from build123d import *

# Parameters (mm, degrees)
CROQUIS1_W                 = 195
CROQUIS1_H                 = 38
CROQUIS1_R                 = 1.625
SALIENTE_EXTRUIR1_DEPTH    = 3
CROQUIS8_W                 = 195
CROQUIS8_H                 = 3
SALIENTE_EXTRUIR5_DEPTH    = 5
CROQUIS9_W                 = 195
CROQUIS9_H                 = 3
SALIENTE_EXTRUIR6_DEPTH    = 5
SALIENTE_EXTRUIR7_START    = -25
SALIENTE_EXTRUIR7_DEPTH    = 35
CROQUIS11_W                = 22.5
CROQUIS11_H                = 8.5
CORTAR_EXTRUIR4_DEPTH      = 24.953943013
CORTAR_EXTRUIR4_DEPTH_BACK = 22.667360251
CORTAR_EXTRUIR5_REACH      = 172
CROQUIS13_R                = 1
CORTAR_EXTRUIR6_DEPTH      = 5
SALIENTE_EXTRUIR8_START    = -25
SALIENTE_EXTRUIR8_DEPTH    = 35
CROQUIS16_W                = 22.5
CROQUIS16_H                = 8.572274099
CORTAR_EXTRUIR7_DEPTH      = 27.836407603
CORTAR_EXTRUIR7_DEPTH_BACK = 17.667360251
CROQUIS17_R                = 1
CORTAR_EXTRUIR8_DEPTH      = 5
CROQUIS18_W                = 35
CROQUIS18_H                = 12
CROQUIS18_R                = 1
CROQUIS18_W_2              = 22.5
CROQUIS18_H_2              = 8.572274099
CROQUIS18_H_3              = 8.5
SALIENTE_EXTRUIR9_DEPTH    = 4


with BuildPart() as part:
    # Croquis1 → Saliente-Extruir1 (new body)
    with BuildSketch(Plane.XY):
        with Locations((0, 19)):
            Rectangle(CROQUIS1_W, CROQUIS1_H)
        with Locations((91.125, 15)):
            Circle(CROQUIS1_R, mode=Mode.SUBTRACT)
        with Locations((-91.125, 15)):
            Circle(CROQUIS1_R, mode=Mode.SUBTRACT)
    extrude(amount=SALIENTE_EXTRUIR1_DEPTH)

    # Croquis8 → Saliente-Extruir5 (add)
    with BuildSketch(Plane.XZ):
        with Locations((0, 1.5)):
            Rectangle(CROQUIS8_W, CROQUIS8_H)
    extrude(amount=SALIENTE_EXTRUIR5_DEPTH)

    # Croquis9 → Saliente-Extruir6 (add)
    with BuildSketch(Plane(origin=(0, 38, 0), x_dir=(1, 0, 0), z_dir=(0, 1, 0))):
        with Locations((0, -1.5)):
            Rectangle(CROQUIS9_W, CROQUIS9_H)
    extrude(amount=SALIENTE_EXTRUIR6_DEPTH)

    # Croquis10 → Saliente-Extruir7 (add)
    with BuildSketch(Plane(origin=(97.5, 0, 0), x_dir=(0, 0, -1), z_dir=(1, 0, 0)).offset(SALIENTE_EXTRUIR7_START)):
        Polygon((0, 39.499839942), (11.100559408, 26.548595056), (1.230032412, 18.088530231), (0, 17.034264947), align=None)
    extrude(amount=-SALIENTE_EXTRUIR7_DEPTH)

    # Croquis11 → Cortar-Extruir4 (cut, two sides)
    with BuildSketch(Plane(origin=(0, 9.820133108, 8.416872039), x_dir=(1, 0, 0), z_dir=(0, -0.759271307, -0.650774217))) as cortar_extruir4_sk:
        with Locations((51.25, -20.45547742)):
            Rectangle(CROQUIS11_W, CROQUIS11_H)
    extrude(amount=CORTAR_EXTRUIR4_DEPTH, mode=Mode.SUBTRACT)
    extrude(cortar_extruir4_sk.sketch, amount=-CORTAR_EXTRUIR4_DEPTH_BACK, mode=Mode.SUBTRACT)

    # Croquis12 → Cortar-Extruir5 (cut, up to next)
    with BuildSketch(Plane(origin=(72.5, 0, 0), x_dir=(0, 0, -1), z_dir=(1, 0, 0)), mode=Mode.PRIVATE) as cortar_extruir5_sk1:
        Polygon((11.100559408, 26.548595056), (0, 17.034264947), (0, 23.619526305), (7.846688321, 30.344951592), align=None)
    cortar_extruir5_tool1 = extrude(cortar_extruir5_sk1.sketch, amount=-CORTAR_EXTRUIR5_REACH, mode=Mode.PRIVATE) & part.part
    add(cortar_extruir5_tool1.solids().sort_by_distance((72.5, 24.238262, -4.783378))[0], mode=Mode.SUBTRACT)

    # Croquis13 → Cortar-Extruir6 (cut)
    with BuildSketch(Plane(origin=(0, 13.616489645, 11.670743125), x_dir=(1, 0, 0), z_dir=(0, -0.759271307, -0.650774217))):
        with Locations((66.25, -20.20547742)):
            Circle(CROQUIS13_R)
    extrude(amount=-CORTAR_EXTRUIR6_DEPTH, mode=Mode.SUBTRACT)

    # Croquis14 → Saliente-Extruir8 (add)
    with BuildSketch(Plane.ZY.offset(97.5).offset(SALIENTE_EXTRUIR8_START)):
        Polygon((0, 23.619526305), (-7.846688321, 30.344951592), (0, 39.499839942), align=None)
    extrude(amount=-SALIENTE_EXTRUIR8_DEPTH)

    # Croquis16 → Cortar-Extruir7 (cut, two sides)
    with BuildSketch(Plane(origin=(0, 13.616489645, 11.670743125), x_dir=(1, 0, 0), z_dir=(0, -0.759271307, -0.650774217))) as cortar_extruir7_sk:
        with Locations((-51.25, -20.491614469)):
            Rectangle(CROQUIS16_W, CROQUIS16_H)
    extrude(amount=CORTAR_EXTRUIR7_DEPTH, mode=Mode.SUBTRACT)
    extrude(cortar_extruir7_sk.sketch, amount=-CORTAR_EXTRUIR7_DEPTH_BACK, mode=Mode.SUBTRACT)

    # Croquis17 → Cortar-Extruir8 (cut)
    with BuildSketch(Plane(origin=(0, 13.616489645, 11.670743125), x_dir=(1, 0, 0), z_dir=(0, -0.759271307, -0.650774217))):
        with Locations((-66.25, -20.20547742)):
            Circle(CROQUIS17_R)
    extrude(amount=-CORTAR_EXTRUIR8_DEPTH, mode=Mode.SUBTRACT)

    # Croquis18 → Saliente-Extruir9 (add)
    with BuildSketch(Plane(origin=(0, 13.616489645, 11.670743125), x_dir=(1, 0, 0), z_dir=(0, -0.759271307, -0.650774217))):
        with Locations((-55, -19.70547742)):
            Rectangle(CROQUIS18_W, CROQUIS18_H)
        with Locations((-66.25, -20.20547742)):
            Circle(CROQUIS18_R, mode=Mode.SUBTRACT)
        with Locations((-51.25, -20.491614469)):
            Rectangle(CROQUIS18_W_2, CROQUIS18_H_2, mode=Mode.SUBTRACT)
        with Locations((55, -19.70547742)):
            Rectangle(CROQUIS18_W, CROQUIS18_H)
        with Locations((66.25, -20.20547742)):
            Circle(CROQUIS18_R, mode=Mode.SUBTRACT)
        with Locations((51.25, -20.45547742)):
            Rectangle(CROQUIS18_W_2, CROQUIS18_H_3, mode=Mode.SUBTRACT)
    extrude(amount=SALIENTE_EXTRUIR9_DEPTH)


solid = part.part
The model under review builds one solid part; all positions refer to its coordinate system, in mm. A direction names the side the tool comes from. Give positions to 0.01 mm unless a question says otherwise; leave off trailing zeros. Order: outer loops, then holes, each group sorted by start corner. A loop starts at its lowest first (then second) coordinate and runs counter-clockwise, first axis right, second up. Notation, with made-up numbers: M -14,29 L 41,29 A17 cw 41,55 Z; hole C -26,-40 d10. An arc over 180 degrees is marked long. Answer in a Markdown table with one row per item. Add a question column.
1. Add section B-B on x = 30.5. State the section outline as (y, z) points.
2. Add section C-C on y = 6. State the section outline as (x, z) points.
3. To check wall thickness, follow line 1 along X through (y, z) = (23, -4.25); line 2 along X through (y, z) = (37, 1.25); line 3 along Z through (x, y) = (78, 38). State the ranges of each line that lie inside material, in increasing order.
4. Add section A-A on y = 15. State the section outline as (x, z) points.
5. Machinability: for faces 1 (the flat face through (-37.5, 27, -4)), 2 (the flat face through (-72.5, 29, -3)), 3 (the flat face through (62.5, 30, -2)), which of the approach directions +Z, -Z, +X, -X, +Y, -Y give a long, thin tool a straight path to every point of the face, cutting with its end or side? Answer none if there is none.
6. Mouldability with a two-part tool opening along Y and no side actions: class faces 4 (the flat face through (54.755, 20.745, -2.793)), 5 (the flat face through (37.5, 29, -3)), 6 (the flat face through (-40, 30, -1)) as released by +Y, released by -Y, zero draft, split by the parting line, or undercut.
7. For pin 1 Ø5 at (y, z) = (27, -5.5) entering from +X; pin 2 Ø6.5 at (y, z) = (35, -5.5) entering from -X; pin 3 Ø3.5 at (x, y) = (-91.125, 15) entering from -Z; pin 4 Ø4 at (x, y) = (91.125, 15) entering from +Z, all flat-tipped, find the tip position at first contact; note any pin that passes through.
The answers:
| question | item | result |
|---|---|---|
| 1 | outline | M -5,0 L 43,0 L 43,3 L -5,3 Z |
| 2 | outline | M -97.5,0 L 97.5,0 L 97.5,3 L -97.5,3 Z |
| 3 | line 1 | -72.5 to -62.5, -40 to -37.5, 37.5 to 40, 62.5 to 72.5 |
| 3 | line 2 | -97.5 to -62.5, -40 to 40, 62.5 to 97.5 |
| 3 | line 3 | 0 to 3 |
| 4 | outline | M -97.5,0 L -92.75,0 L -92.75,3 L -97.5,3 Z; M -89.5,0 L 89.5,0 L 89.5,3 L -89.5,3 Z; M 92.75,0 L 97.5,0 L 97.5,3 L 92.75,3 Z |
| 5 | face 1 | -Z, +Y, -Y |
| 5 | face 2 | -Z, -X, +Y, -Y |
| 5 | face 3 | none |
| 6 | face 4 | released by -Y |
| 6 | face 5 | zero draft |
| 6 | face 6 | undercut |
| 7 | pin 1 | x = 72.5 |
| 7 | pin 2 | x = -72.5 |
| 7 | pin 3 | z = 0 |
| 7 | pin 4 | z = 3 |
